Autodesk Fusion 360 part; units mm, degrees
sketch "Sketch1" plane through (0, 0, 0) normal (0, 1, 0) x (1, 0, 0)
  circle A0 centre (0, 0) radius 30.5 construction
  circle A1 centre (0, -30.5) radius 1.5
  circle A2 centre (0, -30.5) radius 7.5 construction
  line L0 (-7.4123, -31.6434) -> (6.1101, -31.6434) construction
  line L1 (7.4123, -31.6434) -> (22.9663, -31.6434) construction
  line L2 (-7.4123, -31.6434) -> (-3.5355, -27.7667)
  line L3 (7.4123, -31.6434) -> (3.5355, -27.7667)
  arc A3 (3.5355, -27.7667) -> (-3.5355, -27.7667) centre (0, -31.3022) ccw
  circle A4 centre (0, 0) radius 33.5
  arc A5 (27.7667, 3.5355) -> (27.7667, -3.5355) centre (31.3022, 0) ccw
  line L4 (31.6434, -7.4123) -> (27.7667, -3.5355)
  line L5 (31.6434, 7.4123) -> (27.7667, 3.5355)
  circle A6 centre (30.5, 0) radius 1.5
  arc A7 (-3.5355, 27.7667) -> (3.5355, 27.7667) centre (0, 31.3022) ccw
  line L6 (7.4123, 31.6434) -> (3.5355, 27.7667)
  line L7 (-7.4123, 31.6434) -> (-3.5355, 27.7667)
  circle A8 centre (0, 30.5) radius 1.5
  arc A9 (-27.7667, -3.5355) -> (-27.7667, 3.5355) centre (-31.3022, 0) ccw
  line L8 (-31.6434, 7.4123) -> (-27.7667, 3.5355)
  line L9 (-31.6434, -7.4123) -> (-27.7667, -3.5355)
  circle A10 centre (-30.5, 0) radius 1.5
  arc A11 (7.4123, -31.6434) -> (31.6434, -7.4123) centre (0, 0) ccw
  arc A12 (31.6434, 7.4123) -> (7.4123, 31.6434) centre (0, 0) ccw
  arc A13 (-7.4123, 31.6434) -> (-31.6434, 7.4123) centre (0, 0) ccw
  arc A14 (-31.6434, -7.4123) -> (-7.4123, -31.6434) centre (0, 0) ccw
  dimension "d1" = 65
  dimension "d2" = 61
  dimension "d4" = 3
  dimension "d9" = 15
  dimension "d11" = 45
  dimension "d12" = 135
  dimension "d13" = 5
  dimension "d16" = 360
extrude "Extrude1" add sketch "Sketch1" along normal blind 45
sketch "Sketch2" plane through (0, 45, 0) normal (0, 1, 0) x (-1, 0, 0)
  circle A0 centre (-30.5, 0) radius 1.5
  line L0 (31.6434, 7.4123) -> (27.7667, 3.5355)
  arc A1 (27.7667, 3.5355) -> (27.7667, -3.5355) centre (31.3022, 0) ccw
  line L1 (27.7667, -3.5355) -> (31.6434, -7.4123)
  arc A2 (7.4123, -31.6434) -> (31.6434, -7.4123) centre (0, 0) ccw
  line L2 (7.4123, -31.6434) -> (3.5355, -27.7667)
  arc A3 (3.5355, -27.7667) -> (-3.5355, -27.7667) centre (0, -31.3022) ccw
  line L3 (-3.5355, -27.7667) -> (-7.4123, -31.6434)
  arc A4 (-31.6434, -7.4123) -> (-7.4123, -31.6434) centre (0, 0) ccw
  line L4 (-31.6434, -7.4123) -> (-27.7667, -3.5355)
  arc A5 (-27.7667, -3.5355) -> (-27.7667, 3.5355) centre (-31.3022, 0) ccw
  line L5 (-27.7667, 3.5355) -> (-31.6434, 7.4123)
  arc A6 (-7.4123, 31.6434) -> (-31.6434, 7.4123) centre (0, 0) ccw
  line L6 (-7.4123, 31.6434) -> (-3.5355, 27.7667)
  arc A7 (-3.5355, 27.7667) -> (3.5355, 27.7667) centre (0, 31.3022) ccw
  line L7 (3.5355, 27.7667) -> (7.4123, 31.6434)
  arc A8 (31.6434, 7.4123) -> (7.4123, 31.6434) centre (0, 0) ccw
  circle A9 centre (0, 30.5) radius 1.5
  circle A10 centre (0, -30.5) radius 1.5
  circle A11 centre (30.5, 0) radius 1.5
  circle A12 centre (0, 0) radius 33.5
  circle A13 centre (0, 0) radius 33.5
extrude "Extrude2" add sketch "Sketch2" along normal blind 2 contours L0 A1 L1 A2 L2 A3 L3 A4 L4 A5 L5 A6 L6 A7 L7 A8 | A12 A13
Geometry check sheet. Reference: the model listing, model coordinates, mm. Coordinates: 2 decimals unless noted, no trailing zeros. Order: outer loops, then holes, each group sorted by start corner. A loop starts at its lowest first (then second) coordinate and runs counter-clockwise, first axis right, second up. Notation, with made-up numbers: M 49.25,62 L 87.25,62 A25 ccw 87.25,99 Z; hole C -22.5,-6 d4. An arc over 180 degrees is marked long. Answer as a JSON object with one key per item and string values.
Q1. Scan lines: line 1 (Z direction, x = 0, y = 25.5); line 2 (Z direction, x = -30, y = 13.5). Record each from-to range of solid material in increasing order.
Results are:
{"line 1": "z = -33.5 to -32, -29 to -26.3, 26.3 to 29, 32 to 33.5", "line 2": "z = -14.91 to -12.5, -5.77 to -1.41, 1.41 to 5.77, 12.5 to 14.91"}
Q2. Depth check by flat-ended pin: pin 1 Ø2 at (x, z) = (-9.5, -9) entering from -Y; pin 2 Ø8 at (x, y) = (2.5, 25) entering from +Z; pin 3 Ø1 at (y, z) = (13, -12.5) entering from +X. Enter the tip coordinate at first touch or a pass-through.
Results are:
{"pin 1": "stops at y = 45", "pin 2": "stops at z = 33.5", "pin 3": "stops at x = 31.28"}
Q3. Release check for a two-part mould opening along X. For faces 1 (the cylindrical face through (23.16, 22.18, 22.8)), 2 (the flat face through (0, 47, 0)) record: released by +X, released by -X, zero draft, split by the parting line, or undercut.
Results are:
{"face 1": "undercut", "face 2": "zero draft"}
Q4. Cross-section at A-A on y = 40. Record the cut outline in (x, z), and give its area (3 significant figures).
Results are:
{"outline": "C 0,0 d67; hole C -30.5,0 d3; hole M -31.64,-7.41 A32.5 ccw -7.41,-31.64 L -3.54,-27.77 A5 cw 3.54,-27.77 L 7.41,-31.64 A32.5 ccw 31.64,-7.41 L 27.77,-3.54 A5 cw 27.77,3.54 L 31.64,7.41 A32.5 ccw 7.41,31.64 L 3.54,27.77 A5 cw -3.54,27.77 L -7.41,31.64 A32.5 ccw -31.64,7.41 L -27.77,3.54 A5 cw -27.77,-3.54 Z; hole C 0,-30.5 d3; hole C 0,30.5 d3; hole C 30.5,0 d3", "area": "411 mm²"}
